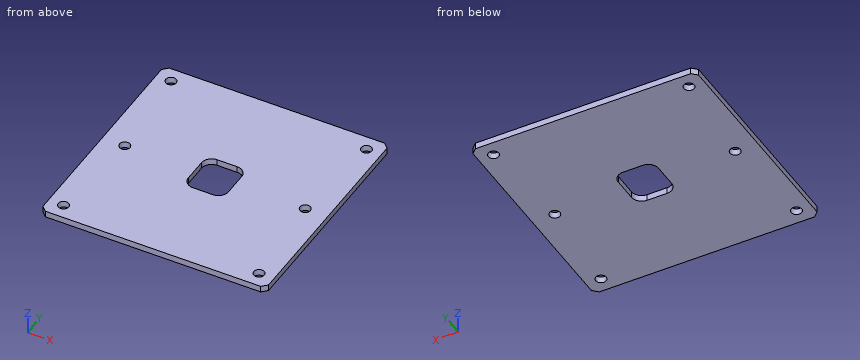
```python
from build123d import *

# Parameters (mm, degrees)
F0_R     = 1.3335
F1_DEPTH = 1.6


with BuildPart() as f1:
    # F0 (on Top) → F1 (new body)
    with BuildSketch(Plane.XY):
        Polygon((55.87, 0), (1.28, 0), (0, -1.28), (0, -55.87), (1.28, -57.15), (55.87, -57.15), (57.15, -55.87), (57.15, -1.28), align=None)
        with Locations((3.81, -53.34)):
            Circle(F0_R, mode=Mode.SUBTRACT)
        with Locations((53.34, -53.34)):
            Circle(F0_R, mode=Mode.SUBTRACT)
        with Locations((5.715, -28.575)):
            Circle(F0_R, mode=Mode.SUBTRACT)
        with Locations((3.81, -3.81)):
            Circle(F0_R, mode=Mode.SUBTRACT)
        with BuildLine():
            ThreePointArc((23.495, -25.527), (24.238949, -23.730949), (26.035, -22.987))
            Line((26.035, -22.987), (31.115, -22.987))
            ThreePointArc((31.115, -22.987), (32.911051, -23.730949), (33.655, -25.527))
            Line((33.655, -25.527), (33.655, -31.623))
            ThreePointArc((33.655, -31.623), (32.911051, -33.419051), (31.115, -34.163))
            Line((31.115, -34.163), (26.035, -34.163))
            ThreePointArc((26.035, -34.163), (24.238949, -33.419051), (23.495, -31.623))
            Line((23.495, -31.623), (23.495, -25.527))
        make_face(mode=Mode.SUBTRACT)
        with Locations((51.435, -28.575)):
            Circle(F0_R, mode=Mode.SUBTRACT)
        with Locations((53.34, -3.81)):
            Circle(F0_R, mode=Mode.SUBTRACT)
    extrude(amount=F1_DEPTH)


solid = f1.part
```
Input: part model. Units: mm. Frame: model coordinates. Coordinates: 2 decimals unless noted, no trailing zeros. Write each loop counter-clockwise with the first axis right and the second up, starting at its lowest first coordinate (ties: lowest second). Pieces come first, ordered by that corner, then holes.
1) Section A-A on y = -53.34. Output: boundary loops of the cut face in (x, z), and give its area (3 significant figures).
2) Material intervals for line 1 along Y through (x, z) = (53.34, 1.15); line 2 along X through (y, z) = (-31, 0.5) (3 decimals); line 3 along Y through (x, z) = (53, 1.45), sorted ascending.
3) Section D-D on z = 0.7. State how many separate pieces and enclosed holes the cut face has, and give its area (3 significant figures).
4) Section B-B on x = 6. Output: boundary loops of the cut face in (y, z), and give its area (3 significant figures).
5) Section C-C on y = -32.5. Output: boundary loops of the cut face in (x, z), and give its area (3 significant figures).
6) Pin query (flat end, axial travel): pin 1 Ø2 at (x, y) = (53.34, -53.34) entering from +Z. Return the tip coordinate at first contact, or that it passes through.
Check result:
1. outline: (0, 0) - (2.48, 0) - (2.48, 1.6) - (0, 1.6) - close; (5.14, 0) - (52.01, 0) - (52.01, 1.6) - (5.14, 1.6) - close; (54.67, 0) - (57.15, 0) - (57.15, 1.6) - (54.67, 1.6) - close
1. area: 82.9 mm2
2. line 1: y = -57.15 to -54.67, -52.01 to -5.14, -2.48 to 0
2. line 2: x = 0 to 23.495, 33.655 to 57.15
2. line 3: y = -57.15 to -54.63, -52.05 to -5.1, -2.52 to 0
3. separate pieces: 1
3. enclosed holes: 7
3. area: 3,120 mm2
4. outline: (-57.15, 0) - (-29.88, 0) - (-29.88, 1.6) - (-57.15, 1.6) - close; (-27.27, 0) - (0, 0) - (0, 1.6) - (-27.27, 1.6) - close
4. area: 87.3 mm2
5. outline: (0, 0) - (23.65, 0) - (23.65, 1.6) - (0, 1.6) - close; (33.5, 0) - (57.15, 0) - (57.15, 1.6) - (33.5, 1.6) - close
5. area: 75.7 mm2
6. pin 1: passes through
